Could you check a few things on this drawing? It's one solid part, dimensions in mm from its lowest x, y, z. A direction names the side the tool comes from. Give positions to 0.01 mm unless a question says otherwise; leave off trailing zeros. Loops run counter-clockwise (first coordinate to the right, second up) from the corner with the lowest first, then second, coordinate; pieces in that order, holes last. Notation, with made-up numbers: (86, 15.5) - (116, 15.5) arc R21 ccw to (116, 51.5) - close; hole circle Ø6 at (72, 70.5). An arc over 180 degrees is marked (long way). Answer as a JSON object with one key per item and string values.
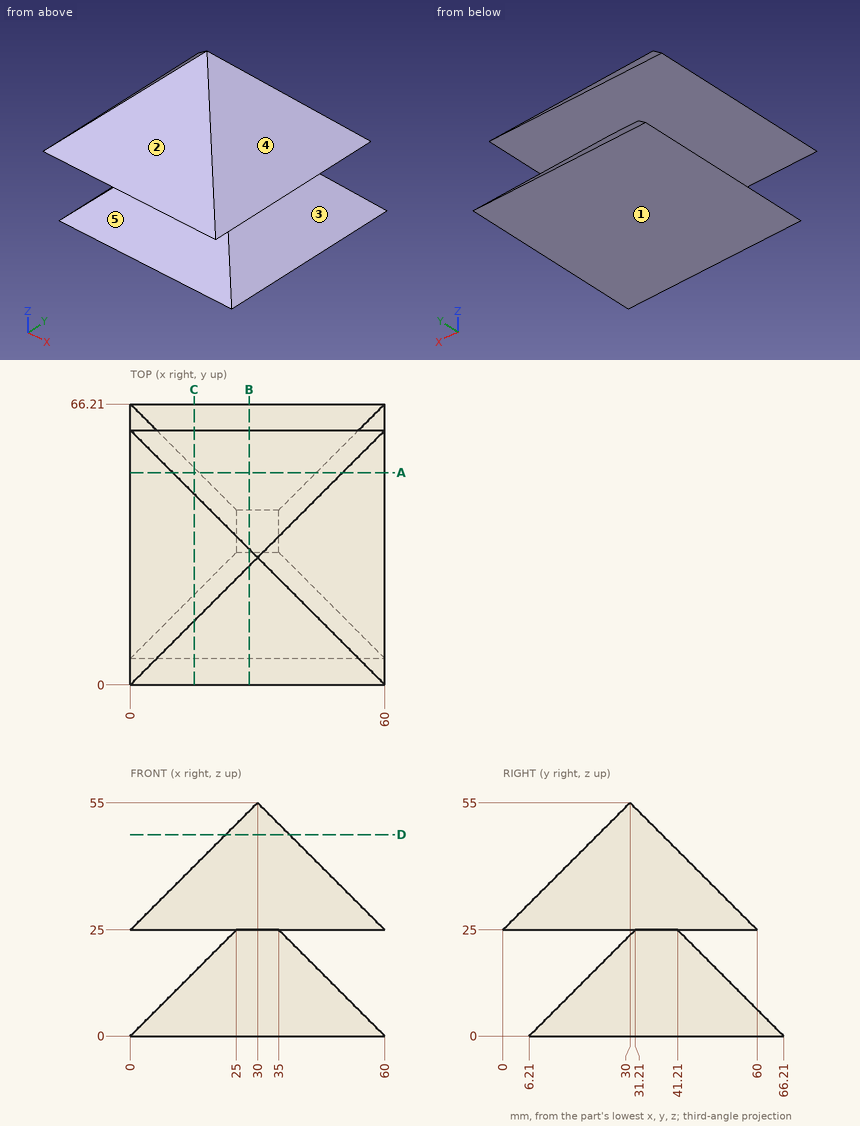
1) If we mould it in two halves opening along Z, with no side actions, what happens to the marked faces 1, 2 and 3? For each: released by +Z, released by -Z, zero draft, split by the parting line, or undercut.
Check sheet entries:
{"face 1": "released by -Z", "face 2": "released by +Z", "face 3": "undercut"}
2) Imagine slicing it at A-A on y = 50. Write out the boundary of the cut face in (x, z), and give its area (3 significant figures).
Check sheet entries:
{"outline": "(0, 0) - (60, 0) - (43.79, 16.21) - (16.21, 16.21) - close; (0, 25) - (60, 25) - (50, 35) - (10, 35) - close", "area": "1,210 mm2"}
3) I'm going to push flat-ended pins straight in: P1, Ø12, axis at y = 13.5, z = 6.5, coming from the +X side; P2, Ø18, axis at x = 44.5, y = 43.5, coming from the -Z side; P3, Ø6, axis at x = 17, z = 38.5, coming from the -Y side; P4, Ø4, axis at x = 19.5, z = 20.5, coming from the -Y side. Where does each tip first touch, or does it pass through?
Check sheet entries:
{"P1": "x = 59.5", "P2": "z = 0", "P3": "y = 10.5", "P4": "y = 24.71"}
4) Which directions (+Z, -Z, +X, -X, +Y, -Y) give clear straight access to the entire face, cutting with the end or side of a thin tool? Please do the marked faces 4 and 5.
Check sheet entries:
{"face 4": "+Z, +X, +Y, -Y", "face 5": "+X, -X, -Y"}
5) I need wall thicknesses on L1, parallel to Z at x = 45, y = 13.5; L2, parallel to Z at x = 52.5, y = 20; L3, parallel to X at y = 43, z = 27.5. Which ranges of each line are inside material? Lowest first, please.
Check sheet entries:
{"L1": "0 to 7.29, 25 to 38.5", "L2": "0 to 7.5, 25 to 32.5", "L3": "2.5 to 57.5"}
6) Imagine slicing it at C-C on x = 15. Write out the boundary of the cut face in (y, z), and give its area (3 significant figures).
Check sheet entries:
{"outline": "(0, 25) - (60, 25) - (45, 40) - (15, 40) - close; (6.21, 0) - (66.21, 0) - (51.21, 15) - (21.21, 15) - close", "area": "1,350 mm2"}
7) Imagine slicing it at D-D on z = 47.5. Write out the boundary of the cut face in (x, y), and give its area (3 significant figures).
Check sheet entries:
{"outline": "(22.5, 22.5) - (37.5, 22.5) - (37.5, 37.5) - (22.5, 37.5) - close", "area": "225 mm2"}
8) Imagine slicing it at B-B on x = 28. Write out the boundary of the cut face in (y, z), and give its area (3 significant figures).
Check sheet entries:
{"outline": "(0, 25) - (31.21, 25) - (6.21, 0) - (66.21, 0) - (41.21, 25) - (60, 25) - (32, 53) - (28, 53) - close", "area": "1,770 mm2"}
